from build123d import *

# Parameters (mm, degrees)
SKETCH1_W               = 132
SKETCH1_H               = 165.15
BOSS_EXTRUDE1_DEPTH     = 6
SKETCH3_W               = 32
SKETCH3_H               = 54
SKETCH3_W_2             = 26
SKETCH3_H_2             = 48
BOSS_EXTRUDE2_DEPTH     = 17.5
SKETCH4_W               = 32
SKETCH4_H               = 54
BOSS_EXTRUDE3_DEPTH     = 3
SKETCH5_W               = 25
SKETCH5_H               = 17
CUT_EXTRUDE1_DEPTH      = 3
SKETCH6_W               = 12
SKETCH6_H               = 54
BOSS_EXTRUDE4_DEPTH     = 3
SKETCH7_R               = 1.6
CUT_EXTRUDE2_DEPTH      = 108.148871319
SKETCH8_W               = 3
SKETCH8_H               = 6.5
BOSS_EXTRUDE5_DEPTH     = 20
SKETCH9_R               = 1.55
CUT_EXTRUDE3_DEPTH      = 6
CUT_EXTRUDE4_DEPTH      = 3
CUT_EXTRUDE4_DEPTH_BACK = 109.981102146
SKETCH10_R              = 1.6
SKETCH10_R_2            = 1.55
SKETCH11_W              = 2.5
SKETCH11_H              = 7
BOSS_EXTRUDE6_DEPTH     = 19.36
SKETCH12_R              = 1.6
CUT_EXTRUDE5_DEPTH      = 19.36
SKETCH13_W              = 3
SKETCH13_H              = 7
BOSS_EXTRUDE7_DEPTH     = 15
SKETCH14_R              = 2
CUT_EXTRUDE6_DEPTH      = 15
CUT_EXTRUDE7_START      = -6
CUT_EXTRUDE7_DEPTH      = 6
SKETCH16_R              = 1.6
CUT_EXTRUDE8_DEPTH      = 15
SKETCH17_W              = 61.848581877
SKETCH17_H              = 62.95797348
CUT_EXTRUDE9_DEPTH      = 52
SKETCH19_R              = 1.55
CUT_EXTRUDE10_DEPTH     = 52
CUT_EXTRUDE11_DEPTH     = 3
SKETCH21_W              = 2.5
SKETCH21_H              = 7
CUT_EXTRUDE12_DEPTH     = 49
SKETCH22_W              = 3
SKETCH22_H              = 7
CUT_EXTRUDE13_DEPTH     = 49
SKETCH22_3_W            = 3
SKETCH22_3_H            = 7
SKETCH22_3_W_2          = 9
CUT_EXTRUDE14_DEPTH     = 3
SKETCH23_R              = 1.55
CUT_EXTRUDE15_DEPTH     = 3
SKETCH26_W              = 3
SKETCH26_H              = 7.6
SKETCH26_W_2            = 3.1
CUT_EXTRUDE17_DEPTH     = 10
SKETCH27_W              = 9.3
SKETCH27_H              = 7.6
SKETCH27_W_2            = 9
CUT_EXTRUDE18_DEPTH     = 3


# Read off the part's stored shape, not the designer's step: Cut-Extrude7
with BuildPart() as part:
    # Sketch1 → Boss-Extrude1 (new body)
    with BuildSketch(Plane.XY):
        Rectangle(SKETCH1_W, SKETCH1_H)
    extrude(amount=BOSS_EXTRUDE1_DEPTH)

    # Sketch3 → Boss-Extrude2 (add)
    with BuildSketch(Plane.XY.offset(6)):
        with Locations((0, -55.575)):
            Rectangle(SKETCH3_W, SKETCH3_H)
        with Locations((0, -55.575)):
            Rectangle(SKETCH3_W_2, SKETCH3_H_2, mode=Mode.SUBTRACT)
    extrude(amount=BOSS_EXTRUDE2_DEPTH)

    # Sketch4 → Boss-Extrude3 (add)
    with BuildSketch(Plane.XY.offset(23.5)):
        with Locations((0, -55.575)):
            Rectangle(SKETCH4_W, SKETCH4_H)
    extrude(amount=BOSS_EXTRUDE3_DEPTH)

    # Sketch5 → Cut-Extrude1 (cut)
    with BuildSketch(Plane.XZ.offset(82.575)):
        with Locations((0, 14.5)):
            Rectangle(SKETCH5_W, SKETCH5_H)
    extrude(amount=-CUT_EXTRUDE1_DEPTH, mode=Mode.SUBTRACT)

    # Sketch6 → Boss-Extrude4 (add)
    with BuildSketch(Plane.XY.offset(6)):
        with Locations((-22, -55.575)):
            Rectangle(SKETCH6_W, SKETCH6_H)
        with Locations((22, -55.575)):
            Rectangle(SKETCH6_W, SKETCH6_H)
    extrude(amount=BOSS_EXTRUDE4_DEPTH)

    # Sketch7 → Cut-Extrude2 (cut, through all)
    with BuildSketch(Plane.XY.offset(9)):
        with Locations((-22, -69.005)):
            Circle(SKETCH7_R)
        with Locations((-22, -33.005)):
            Circle(SKETCH7_R)
        with Locations(Location((22, -69.005, 0), (0, 0, 180))):
            Circle(SKETCH7_R)
        with Locations(Location((22, -33.005, 0), (0, 0, 180))):
            Circle(SKETCH7_R)
    extrude(amount=-CUT_EXTRUDE2_DEPTH, mode=Mode.SUBTRACT)

    # Sketch8 → Boss-Extrude5 (add)
    with BuildSketch(Plane.XY.offset(6)):
        with Locations((-54.38, -79.325)):
            Rectangle(SKETCH8_W, SKETCH8_H)
        with Locations((-54.38, -31.825)):
            Rectangle(SKETCH8_W, SKETCH8_H)
    boss_extrude5 = extrude(amount=BOSS_EXTRUDE5_DEPTH)

    # Sketch9 → Cut-Extrude3 (cut)
    with BuildSketch(Plane.ZY.offset(55.88)):
        with Locations((10.5, -79.325)):
            Circle(SKETCH9_R)
        with Locations((20.8, -79.325)):
            Circle(SKETCH9_R)
        with Locations((10.5, -31.825)):
            Circle(SKETCH9_R)
        with Locations((20.8, -31.825)):
            Circle(SKETCH9_R)
    cut_extrude3 = extrude(amount=-CUT_EXTRUDE3_DEPTH, mode=Mode.SUBTRACT)

    # Mirror1: Boss-Extrude5, Cut-Extrude3 across plane
    add(boss_extrude5.mirror(Plane(origin=(0, 0, 0), x_dir=(0, 0, 1), z_dir=(1, 0, 0))))
    add(cut_extrude3.mirror(Plane(origin=(0, 0, 0), x_dir=(0, 0, 1), z_dir=(1, 0, 0))), mode=Mode.SUBTRACT)

    # Sketch10 → Cut-Extrude4 (cut, two sides: drawn at the far end of the back side and taken through both)
    with BuildSketch(Plane(origin=(0, 0, 0), x_dir=(-1, 0, 0), z_dir=(0, 0, -1)).offset(-CUT_EXTRUDE4_DEPTH_BACK)):
        with Locations(Location((-24.1, -75.572749788, 0), (0, 0, 180))):
            Circle(SKETCH10_R)
        with Locations(Location((-20.925, -9.532749788, 0), (0, 0, 180))):
            Circle(SKETCH10_R_2)
        with Locations(Location((20.925, -9.532749788, 0), (0, 0, 180))):
            Circle(SKETCH10_R_2)
        with Locations(Location((24.1, -75.572749788, 0), (0, 0, 180))):
            Circle(SKETCH10_R)
    extrude(amount=CUT_EXTRUDE4_DEPTH + CUT_EXTRUDE4_DEPTH_BACK, mode=Mode.SUBTRACT)

    # Sketch11 → Boss-Extrude6 (add)
    with BuildSketch(Plane(origin=(0, 0, 0), x_dir=(-1, 0, 0), z_dir=(0, 0, -1))):
        with Locations((-17.675, 4.467250212)):
            Rectangle(SKETCH11_W, SKETCH11_H)
        with Locations((-17.675, 53.467250212)):
            Rectangle(SKETCH11_W, SKETCH11_H)
    extrude(amount=BOSS_EXTRUDE6_DEPTH)

    # Sketch12 → Cut-Extrude5 (cut)
    with BuildSketch(Plane(origin=(18.925, 0, 0), x_dir=(0, 0, -1), z_dir=(1, 0, 0))):
        with Locations(Location((4.5, 53.467250212, 0), (0, 0, 90))):
            Circle(SKETCH12_R)
        with Locations(Location((14.5, 53.467250212, 0), (0, 0, 90))):
            Circle(SKETCH12_R)
        with Locations(Location((4.5, 4.467250212, 0), (0, 0, 90))):
            Circle(SKETCH12_R)
        with Locations(Location((14.5, 4.467250212, 0), (0, 0, 90))):
            Circle(SKETCH12_R)
    extrude(amount=-CUT_EXTRUDE5_DEPTH, mode=Mode.SUBTRACT)

    # Sketch13 → Boss-Extrude7 (add)
    with BuildSketch(Plane(origin=(0, 0, 0), x_dir=(-1, 0, 0), z_dir=(0, 0, -1))):
        with Locations((29.575, 39.167250212)):
            Rectangle(SKETCH13_W, SKETCH13_H)
    extrude(amount=BOSS_EXTRUDE7_DEPTH)

    # Sketch14 → Cut-Extrude6 (cut)
    with BuildSketch(Plane.ZY.offset(31.075)):
        with Locations((-9.9, 39.167250212)):
            Circle(SKETCH14_R)
    extrude(amount=-CUT_EXTRUDE6_DEPTH, mode=Mode.SUBTRACT)

    # Cut-Extrude7 outline → Cut-Extrude7 (cut)
    with BuildSketch(Plane(origin=(0, 0, 0), x_dir=(-1, 0, 0), z_dir=(0, 0, -1)).offset(CUT_EXTRUDE7_START)):
        Polygon((-31.075, 59.967250212), (31.075, 59.967250212), (31.075, -24), (58.88, -24), (58.88, -82.575), (66, -82.575), (66, 82.575), (-66, 82.575), (-66, -82.575), (-58.88, -82.575), (-58.88, -24), (-31.075, -24), align=None)
    extrude(amount=CUT_EXTRUDE7_DEPTH, mode=Mode.SUBTRACT)

    # Sketch16 → Cut-Extrude8 (cut)
    with BuildSketch(Plane(origin=(0, 0, 0), x_dir=(-1, 0, 0), z_dir=(0, 0, -1))):
        Circle(SKETCH16_R)
        with Locations((0, 55.967250212)):
            Circle(SKETCH16_R)
    extrude(amount=-CUT_EXTRUDE8_DEPTH, mode=Mode.SUBTRACT)

    # Sketch17 → Cut-Extrude9 (cut)
    with BuildSketch(Plane.XY.offset(6)):
        with Locations((1.152470824, -55.437355719)):
            Rectangle(SKETCH17_W, SKETCH17_H)
    extrude(amount=CUT_EXTRUDE9_DEPTH, mode=Mode.SUBTRACT)

    # Sketch19 → Cut-Extrude10 (cut)
    with BuildSketch(Plane.XY.offset(6)):
        with Locations((24.425, 4.467250212)):
            Circle(SKETCH19_R)
    cut_extrude10 = extrude(amount=-CUT_EXTRUDE10_DEPTH, mode=Mode.SUBTRACT)

    # Sketch19<3> → Cut-Extrude11 (cut)
    with BuildSketch(Plane.XY.offset(6)):
        Polygon((18.925, 0.967250212), (16.425, 0.967250212), (16.425, 7.967250212), (18.925, 7.967250212), (27.925, 7.967250212), (27.925, 0.967250212), align=None)
    cut_extrude11 = extrude(amount=-CUT_EXTRUDE11_DEPTH, mode=Mode.SUBTRACT)

    # Sketch21 → Cut-Extrude12 (cut)
    with BuildSketch(Plane(origin=(0, 0, -19.36), x_dir=(-1, 0, 0), z_dir=(0, 0, -1))):
        with Locations((-17.675, 4.467250212)):
            Rectangle(SKETCH21_W, SKETCH21_H)
    cut_extrude12 = extrude(amount=-CUT_EXTRUDE12_DEPTH, mode=Mode.SUBTRACT)

    # Mirror2: Cut-Extrude10, Cut-Extrude11, Cut-Extrude12 across plane
    add(cut_extrude10.mirror(Plane(origin=(0, 28.967250212, 0), x_dir=(0, 0, 1), z_dir=(0, -1, 0))), mode=Mode.SUBTRACT)
    add(cut_extrude11.mirror(Plane(origin=(0, 28.967250212, 0), x_dir=(0, 0, 1), z_dir=(0, -1, 0))), mode=Mode.SUBTRACT)
    add(cut_extrude12.mirror(Plane(origin=(0, 28.967250212, 0), x_dir=(0, 0, 1), z_dir=(0, -1, 0))), mode=Mode.SUBTRACT)

    # Sketch22 → Cut-Extrude13 (cut)
    with BuildSketch(Plane.XY.offset(6)):
        with Locations((-29.575, 39.167250212)):
            Rectangle(SKETCH22_W, SKETCH22_H)
    extrude(amount=-CUT_EXTRUDE13_DEPTH, mode=Mode.SUBTRACT)

    # Sketch22<3> → Cut-Extrude14 (cut)
    with BuildSketch(Plane.XY.offset(6)):
        with Locations((-29.575, 39.167250212)):
            Rectangle(SKETCH22_3_W, SKETCH22_3_H)
        with Locations((-23.575, 39.167250212)):
            Rectangle(SKETCH22_3_W_2, SKETCH22_3_H)
    extrude(amount=-CUT_EXTRUDE14_DEPTH, mode=Mode.SUBTRACT)

    # Sketch23 → Cut-Extrude15 (cut)
    with BuildSketch(Plane.XY.offset(3)):
        with Locations((-22.575, 39.167250212)):
            Circle(SKETCH23_R)
    extrude(amount=-CUT_EXTRUDE15_DEPTH, mode=Mode.SUBTRACT)

    # Sketch26 → Cut-Extrude17 (cut)
    with BuildSketch(Plane(origin=(0, 0, 0), x_dir=(-1, 0, 0), z_dir=(0, 0, -1))):
        with Locations((29.575, 39.167250212)):
            Rectangle(SKETCH26_W, SKETCH26_H)
        with Locations((-17.675, 53.467250212)):
            Rectangle(SKETCH26_W_2, SKETCH26_H)
        with Locations((-17.675, 4.467250212)):
            Rectangle(SKETCH26_W_2, SKETCH26_H)
    extrude(amount=-CUT_EXTRUDE17_DEPTH, mode=Mode.SUBTRACT)

    # Sketch27 → Cut-Extrude18 (cut)
    with BuildSketch(Plane.XY.offset(6)):
        with Locations((-23.425, 39.167250212)):
            Rectangle(SKETCH27_W, SKETCH27_H)
        with Locations((23.725, 4.467250212)):
            Rectangle(SKETCH27_W_2, SKETCH27_H)
        with Locations((23.575, 53.467250212)):
            Rectangle(SKETCH27_W, SKETCH27_H)
    extrude(amount=-CUT_EXTRUDE18_DEPTH, mode=Mode.SUBTRACT)


solid = part.part
Verification items for the finished model (mm, model axes). A direction names the side the tool comes from. Coordinates: 2 decimals unless noted, no trailing zeros. Order: outer loops, then holes, each group sorted by start corner. A loop starts at its lowest first (then second) coordinate and runs counter-clockwise, first axis right, second up. Notation, with made-up numbers: (53.25, 2) -> (105.25, 2) arc R33 cw to (105.25, 30) -> close; hole circle Ø9 at (62, 15). An arc over 180 degrees is marked (long way). Use CSV: the item, a comma, the result in double quotes. Start each with the question number.
Q1. Section check D-D, the plane x = 49. Record the cut outline in (y, z) (3 decimals).
Q2. Depth check by flat-ended pin: P1, Ø3, axis at y = -79.325, z = 20.8, coming from the -X side; P2, Ø5, axis at x = -24.1, y = -75.57, coming from the +Z side; P3, Ø0.9, axis at y = 40.5, z = 1, coming from the -X side (3 decimals); P4, Ø2, axis at y = -30.5, z = 16, coming from the +X side. Enter the tip coordinate at first touch or a pass-through.
Q3. Section check A-A, the plane z = 13.75. Record the cut outline in (x, y) (3 decimals), and give its area (3 significant figures).
Q4. Section check B-B, the plane x = 0. Record the cut outline in (y, z) (3 decimals).
Q5. Tool access check on faces 1 (the flat face through (-18.775, 39, 5)), 2 (the flat face through (52.88, -79, 16)), 3 (the flat face through (19.225, 4, 1)), 4 (the flat face through (-45, -24, 3)), 5 (the flat face through (22.7, 53.5, 3)). Record the directions out of +Z, -Z, +X, -X, +Y, -Y that give a thin tool (end or side, any length) a straight path to the whole face; none if there is none.
Q6. Section check C-C, the plane y = -20. Record the cut outline in (x, z) (3 decimals).
Q7. Thickness scan on line 1 along Y through (x, z) = (-54.25, 20.8) (3 decimals); line 2 along X through (y, z) = (-29, 15.75); line 3 along X through (y, z) = (53.5, 3.75) (3 decimals). Record the ranges inside material, lowest first.
Q8. Draft check along X on faces 6 (the cylindrical face through (-54.4, -80.27, 9.27)), 7 (the flat face through (-28.075, 39, 1)), 8 (the cylindrical face through (21.262, -31.586, 3.042)). Enter one of: +X half, -X half, draft (parallel to the pull), parting line (faces both ways), or undercut.
Returned:
1,outline,"(-82.575, 0) -> (-24, 0) -> (-24, 6) -> (-82.575, 6) -> close"
2,P1,"passes through"
2,P2,"stops at z = 6"
2,P3,"stops at x = -28.075"
2,P4,"stops at x = 55.88"
3,outline,"(-55.88, -82.575) -> (-52.88, -82.575) -> (-52.88, -76.075) -> (-55.88, -76.075) -> close; (-55.88, -35.075) -> (-52.88, -35.075) -> (-52.88, -28.575) -> (-55.88, -28.575) -> close; (52.88, -82.575) -> (55.88, -82.575) -> (55.88, -76.075) -> (52.88, -76.075) -> close; (52.88, -35.075) -> (55.88, -35.075) -> (55.88, -28.575) -> (52.88, -28.575) -> close"
3,area,"78.0 mm^2"
4,outline,"(-82.575, 0) -> (-1.6, 0) -> (-1.6, 6) -> (-82.575, 6) -> close; (1.6, 0) -> (54.367, 0) -> (54.367, 6) -> (1.6, 6) -> close; (57.567, 0) -> (59.967, 0) -> (59.967, 6) -> (57.567, 6) -> close"
5,face 1,"+Z, -X"
5,face 2,"+Z, +Y, -Y"
5,face 3,"+Z, -Z"
5,face 4,"+Z, -Z, -X, +Y"
5,face 5,"+Z"
6,outline,"(-31.075, 0) -> (31.075, 0) -> (31.075, 6) -> (-31.075, 6) -> close"
7,line 1,"y = -82.575 to -80.875, -77.775 to -76.075, -35.075 to -33.375, -30.275 to -28.575"
7,line 2,"x = -55.88 to -52.88, 52.88 to 55.88"
7,line 3,"x = -31.075 to 16.125, 28.225 to 31.075"
8,face 6,"draft"
8,face 7,"-X half"
8,face 8,"undercut"
